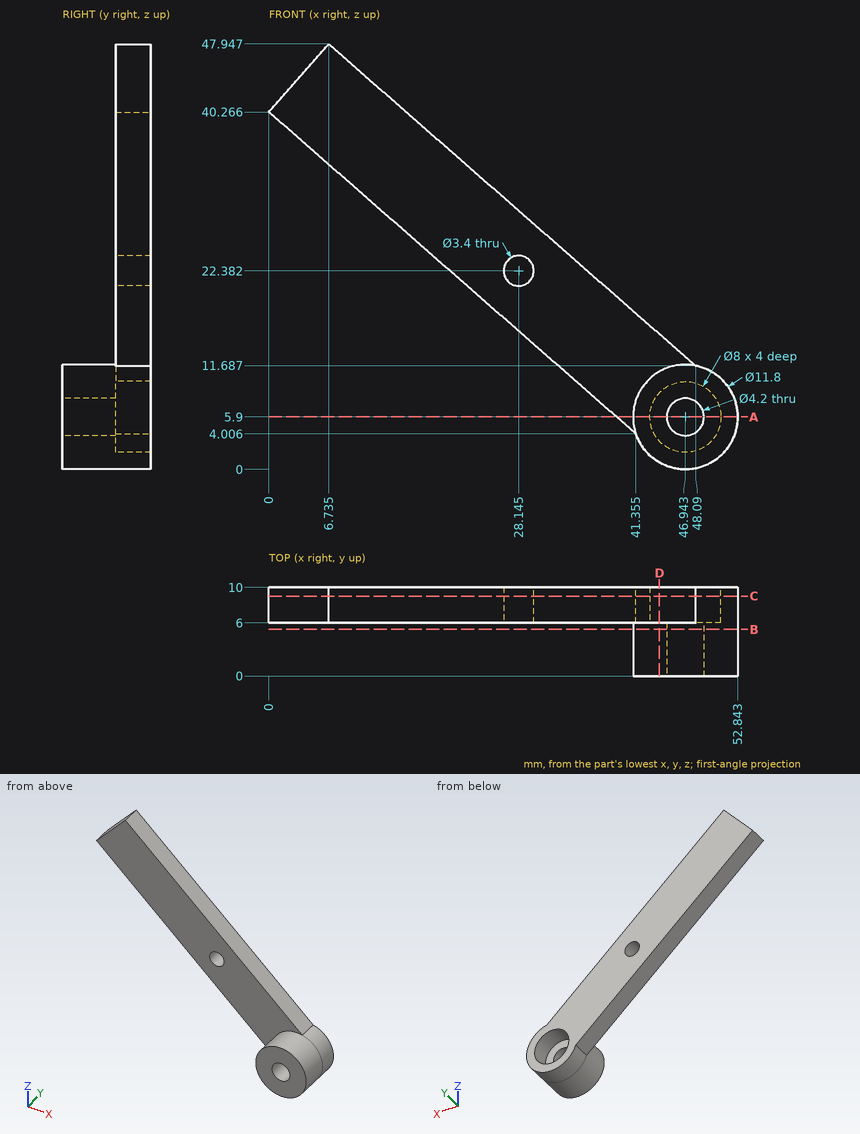
For this review, use the dimensioned drawing (mm, ordinates from the lowest corner) and the shaded views. Coordinates: 2 decimals unless noted, no trailing zeros. Order: outer loops, then holes, each group sorted by start corner. A loop starts at its lowest first (then second) coordinate and runs counter-clockwise, first axis right, second up. Notation, with made-up numbers: (-26.5, 64.25) - (-20.5, 64.25) arc R21 ccw to (-20.5, 93.25) - close; hole circle Ø11 at (77, 29.25). An arc over 180 degrees is marked (long way). Use one line per item in the form item = value.
Q1. Consider section D-D (x = 44). Give the boundary of the cut face in (y, z).
Checked values:
outline = (0, 0.79) - (10, 0.79) - (10, 3.19) - (6, 3.19) - (6, 8.61) - (10, 8.61) - (10, 15.27) - (6, 15.27) - (6, 11.01) - (0, 11.01) - close
Q2. Consider section A-A (z = 5.9). Give the boundary of the cut face in (x, y) (1 decimal).
Checked values:
outline = (39.2, 6) - (41, 6) - (41, 0) - (44.8, 0) - (44.8, 6) - (42.9, 6) - (42.9, 10) - (39.2, 10) - close; (49, 0) - (52.8, 0) - (52.8, 10) - (50.9, 10) - (50.9, 6) - (49, 6) - close
Q3. For probe 1 along Y at (x, z) = (19.5, 31.5); probe 2 along Z at (x, y) = (48.5, 2.25); probe 3 along Z at (x, y) = (44.5, 8) (1 decimal), list the stretches that pass through material, from the lowest coordinate up. Write a range as from..to.
Checked values:
probe_1 = 6..10
probe_2 = 0.21..4.49, 7.31..11.59
probe_3 = 0.5..2.7, 9.1..14.8
Q4. For P1, Ø2, axis at y = 4.5, z = 21, coming from the +X side; P2, Ø4, axis at x = 11, z = 30, coming from the -Y side; P3, Ø4, axis at x = 32.5, y = 8.5, coming from the +Z side; P4, Ø4, axis at x = 13, y = 7, coming from the -Z side (1 decimal), all flat-tipped, find the tip position at first contact; note any pin that passes through.
Checked values:
P1 = through
P2 = 6
P3 = 27.11
P4 = 27.1
Q5. Consider section B-B (y = 5.25). Give the boundary of the cut face in (x, z) (1 decimal).
Checked values:
outline = circle Ø11.8 at (46.9, 5.9); hole circle Ø4.2 at (46.9, 5.9)
Q6. Consider section C-C (y = 9). Give the boundary of the cut face in (x, z) (1 decimal).
Checked values:
outline = (0, 40.3) - (41.4, 4) arc R5.9 ccw (long way) to (48.1, 11.7) - (6.7, 47.9) - close; hole circle Ø3.4 at (28.1, 22.4); hole circle Ø8 at (46.9, 5.9)
